The drawing under review shows one solid part. Ordinate dimensions are in mm from its lowest x, y, z. A direction names the side the tool comes from. Give positions to 0.01 mm unless a question says otherwise; leave off trailing zeros. Loops run counter-clockwise (first coordinate to the right, second up) from the corner with the lowest first, then second, coordinate; pieces in that order, holes last.
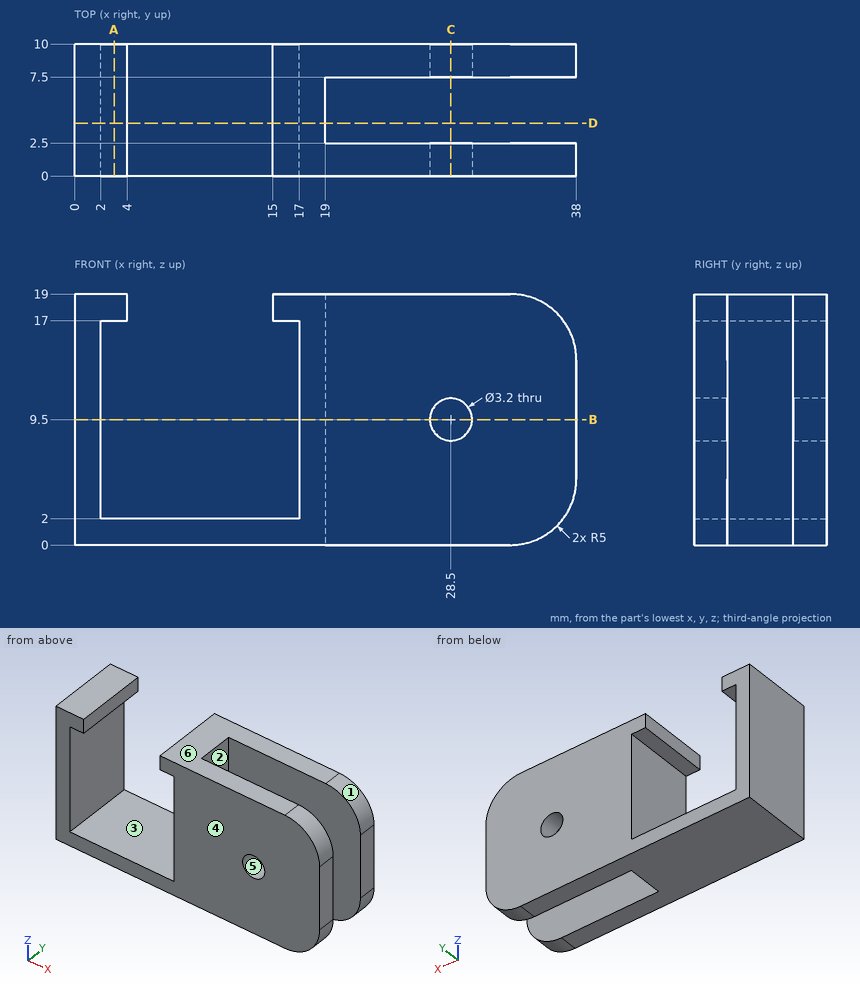
Item 1: Take a section at B-B on z = 9.5. Give the boundary of the cut face in (x, y), and give its area (3 significant figures).
Answer:
outline: (0, 0) - (2, 0) - (2, 10) - (0, 10) - close; (17, 0) - (26.9, 0) - (26.9, 2.5) - (19, 2.5) - (19, 7.5) - (26.9, 7.5) - (26.9, 10) - (17, 10) - close; (30.1, 0) - (38, 0) - (38, 2.5) - (30.1, 2.5) - close; (30.1, 7.5) - (38, 7.5) - (38, 10) - (30.1, 10) - close
area: 119 mm2
Item 2: The part is to be moulded in two halves that separate along Z. For the marked faces 4, 5 and 6, say which applies: released by +Z, released by -Z, zero draft, split by the parting line, or undercut.
Answer:
face 4: zero draft
face 5: undercut
face 6: released by +Z
Item 3: Take a section at D-D on y = 4. Give the boundary of the cut face in (x, z), and give its area (3 significant figures).
Answer:
outline: (0, 0) - (19, 0) - (19, 19) - (15, 19) - (15, 17) - (17, 17) - (17, 2) - (2, 2) - (2, 17) - (4, 17) - (4, 19) - (0, 19) - close
area: 114 mm2
Item 4: Take a section at A-A on x = 3. Give the boundary of the cut face in (y, z).
Answer:
outline: (0, 0) - (10, 0) - (10, 2) - (0, 2) - close; (0, 17) - (10, 17) - (10, 19) - (0, 19) - close
Item 5: For L1, parallel to X at y = 1.15, z = 9.5; L2, parallel to Y at x = 29, z = 12.5; L3, parallel to X at y = 5, z = 14, list the stretches that pass through material, from the lowest coordinate up.
Answer:
L1: x = 0 to 2, 17 to 26.9, 30.1 to 38
L2: y = 0 to 2.5, 7.5 to 10
L3: x = 0 to 2, 17 to 19
Item 6: Tool access review of the marked faces 1, 2 and 3: name each direction out of +Z, -Z, +X, -X, +Y, -Y from which nothing blocks a thin tool from reaching the whole face with its end or side.
Answer:
face 1: +Z, +X, +Y, -Y
face 2: +Z, -Z, +X
face 3: +Y, -Y
Item 7: Take a section at C-C on x = 28.5. Give the boundary of the cut face in (y, z).
Answer:
outline: (0, 0) - (2.5, 0) - (2.5, 7.9) - (0, 7.9) - close; (0, 11.1) - (2.5, 11.1) - (2.5, 19) - (0, 19) - close; (7.5, 0) - (10, 0) - (10, 7.9) - (7.5, 7.9) - close; (7.5, 11.1) - (10, 11.1) - (10, 19) - (7.5, 19) - close
Item 8: Clearance check with flat-ended pins moving along their axes: pin 1 Ø4 at (x, z) = (12.5, 5) entering from +Y (3 decimals); pin 2 Ø1.5 at (x, y) = (6.5, 7) entering from +Z; pin 3 Ø0.6 at (y, z) = (6.5, 18) entering from +X; pin 4 Ø1 at (y, z) = (1, 15) entering from +X. State where each tip first meets the part, or that it passes through.
Answer:
pin 1: passes through
pin 2: stops at z = 2
pin 3: stops at x = 19
pin 4: stops at x = 37.97
